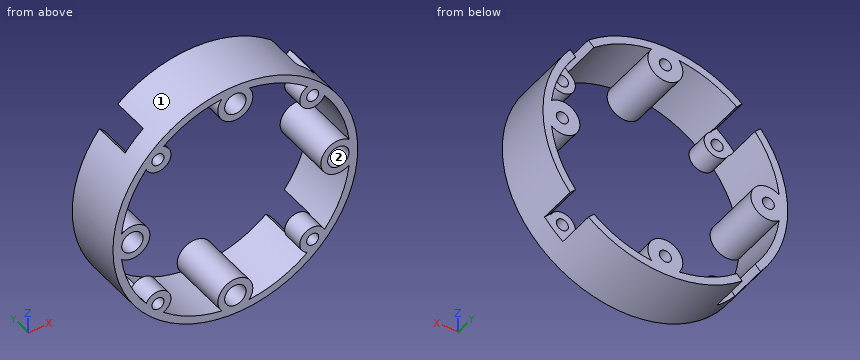
Autodesk Inventor part; units mm, degrees
ref_plane "YZ Plane" through (0, 0, 0) normal (1, 0, 0) x (0, 1, 0)
ref_plane "XZ Plane" through (0, 0, 0) normal (0, 1, 0) x (-1, 0, 0)
ref_plane "XY Plane" through (0, 0, 0) normal (0, 0, 1) x (1, 0, 0)
sketch "Sketch1" plane through (0, 0, 0) normal (0, 1, 0) x (-1, 0, 0)
  circle A0 centre (0, 0) radius 31.5
  circle A1 centre (0, 0) radius 29.5
  dimension "d0" = 63
  dimension "d1" = 59
extrude "Walls" add sketch "Sketch1" along normal blind 15.9
sketch "Sketch2" plane through (0, 0, 0) normal (0, -1, 0) x (1, 0, 0)
  circle A0 centre (0, 0) radius 31.5
  line L0 (0, -31.5) -> (0, -26.5)
  circle A1 centre (0, -26.5) radius 2.75
  circle A2 centre (0, -26.5) radius 4.5
  circle A3 centre (26.5, 0) radius 4.5
  circle A4 centre (26.5, 0) radius 2.75
  circle A5 centre (0, 26.5) radius 4.5
  circle A6 centre (0, 26.5) radius 2.75
  circle A7 centre (-26.5, 0) radius 4.5
  circle A8 centre (-26.5, 0) radius 2.75
  dimension "d4" = 5
  dimension "d5" = 5.5
  dimension "d6" = 9
  dimension "d9" = 360
extrude "Pillar holes" add sketch "Sketch2" against normal blind 15.9 contours A2 | A3 | A5 | A7
sketch "Sketch4" plane through (0, 15.9, 0) normal (0, 1, 0) x (1, 0, 0)
  point P0 (0, 0)
sketch "Sketch5" plane through (0, 0, 0) normal (0, -1, 0) x (1, 0, 0)
  point P0 (0, 0)
sketch "Sketch6" plane through (0, 15.9, 0) normal (0, 1, 0) x (1, 0, 0)
  circle A0 centre (0, 26.5) radius 2.75
  circle A1 centre (0, 26.5) radius 2.75
  circle A2 centre (0, 26.5) radius 1.55
  circle A3 centre (-26.5, 0) radius 1.55
  circle A4 centre (-26.5, 0) radius 2.75
  circle A5 centre (0, -26.5) radius 1.55
  circle A6 centre (0, -26.5) radius 2.75
  circle A7 centre (26.5, 0) radius 1.55
  circle A8 centre (26.5, 0) radius 2.75
  point P0 (0, 0)
  dimension "d20" = 3.1
  dimension "d23" = 360
extrude "Extrusion4" add sketch "Sketch6" against normal blind 8
sketch "Sketch7" plane through (0, 15.9, 0) normal (0, 1, 0) x (1, 0, 0)
  line L0 (0, 0) -> (22.2739, -22.2739)
  circle A0 centre (0, 0) radius 31.5
  line L1 (0, 0) -> (0, -31.5)
  line L2 (0, 0) -> (-22.2739, -22.2739)
  dimension "d27" = 45
ref_plane "Work Plane1" through (22.2739, 15.9, 22.2739) normal (0.7071, 0, 0.7071) x (0, 1, 0)
ref_plane "Work Plane2" through (-22.2739, 15.9, 22.2739) normal (-0.7071, 0, 0.7071) x (0, -1, 0)
sketch "Sketch17" plane through (0, 15.9, 0) normal (0, 1, 0) x (1, 0, 0)
  line L0 (0, 0) -> (-22.2739, -22.2739)
  line L1 (0, 0) -> (0, -14.1086)
  line L2 (-22.2739, -22.2739) -> (-19.9135, -19.9135)
  circle A0 centre (-19.9135, -19.9135) radius 1.55
  circle A1 centre (-19.9135, -19.9135) radius 3.338
  circle A2 centre (19.9135, -19.9135) radius 1.55
  circle A3 centre (19.9135, -19.9135) radius 3.338
  circle A4 centre (19.9135, 19.9135) radius 1.55
  circle A5 centre (19.9135, 19.9135) radius 3.338
  circle A6 centre (-19.9135, 19.9135) radius 1.55
  circle A7 centre (-19.9135, 19.9135) radius 3.338
  point P0 (22.2739, -22.2739)
  point P1 (22.2739, 22.2739)
  point P2 (-22.2739, 22.2739)
  dimension "d86" = 31.5
  dimension "d87" = 45
  dimension "d88" = 3.338
  dimension "d89" = 3.1
  dimension "d92" = 360
extrude "Extrusion13" add sketch "Sketch17" against normal blind 15.9 contours A1 L0 A0 | L0 A0 A1 | A0 L0 | L0 A0 | A2 | A3 | A4 | A5 | A6 | A7
sketch "Sketch18" plane through (0, 15.9, 0) normal (0, 1, 0) x (1, 0, 0)
  circle A0 centre (0, 0) radius 31.5
  line L0 (0, 0) -> (-22.2739, -22.2739)
  line L1 (0, 0) -> (0, -10.409)
  line L2 (-22.2739, -22.2739) -> (-19.9135, -19.9135)
  circle A1 centre (-19.9135, -19.9135) radius 1.55
  circle A2 centre (19.9135, -19.9135) radius 1.55
  circle A3 centre (19.9135, 19.9135) radius 1.55
  circle A4 centre (-19.9135, 19.9135) radius 1.55
  dimension "d96" = 45
  dimension "d97" = 3.338
  dimension "d98" = 3.1
  dimension "d101" = 360
extrude "Extrusion14" cut sketch "Sketch18" against normal blind 15.9 contours A1 L0 | L0 A1 | A2 | A3 | A4
sketch "Sketch19" plane through (0, 15.9, 0) normal (0, 1, 0) x (1, 0, 0)
  arc A0 (22.9523, -18.5322) -> (18.5322, -22.9523) centre (19.9135, -19.9135) ccw
  circle A1 centre (19.9135, -19.9135) radius 3.338
  circle A2 centre (19.9135, -19.9135) radius 1.55
  line L0 (19.9135, -19.9135) -> (17.5532, -22.2739)
  line L1 (19.9135, -19.9135) -> (22.2739, -17.5532)
  line L2 (17.5532, -22.2739) -> (19.7881, -24.5088)
  circle A3 centre (0, 0) radius 31.5
  line L3 (22.2739, -17.5532) -> (24.5088, -19.7881)
  line L4 (17.5532, -17.5532) -> (19.9135, -15.1929)
  line L5 (19.9135, -15.1929) -> (22.2739, -17.5532)
  line L6 (17.5532, -17.5532) -> (15.1929, -19.9135)
  line L7 (15.1929, -19.9135) -> (17.5532, -22.2739)
  arc A4 (19.7881, -24.5088) -> (24.5088, -19.7881) centre (0, 0) ccw
  line L8 (19.9135, 15.1929) -> (22.2739, 17.5532)
  line L9 (22.2739, 17.5532) -> (24.5088, 19.7881)
  arc A5 (24.5088, 19.7881) -> (19.7881, 24.5088) centre (0, 0) ccw
  circle A6 centre (19.9135, 19.9135) radius 3.338
  line L10 (17.5532, 17.5532) -> (15.1929, 19.9135)
  line L11 (17.5532, 17.5532) -> (19.9135, 15.1929)
  line L12 (15.1929, 19.9135) -> (17.5532, 22.2739)
  line L13 (17.5532, 22.2739) -> (19.7881, 24.5088)
  line L14 (-15.1929, 19.9135) -> (-17.5532, 22.2739)
  line L15 (-17.5532, 22.2739) -> (-19.7881, 24.5088)
  arc A7 (-19.7881, 24.5088) -> (-24.5088, 19.7881) centre (0, 0) ccw
  circle A8 centre (-19.9135, 19.9135) radius 3.338
  line L16 (-17.5532, 17.5532) -> (-19.9135, 15.1929)
  line L17 (-17.5532, 17.5532) -> (-15.1929, 19.9135)
  line L18 (-19.9135, 15.1929) -> (-22.2739, 17.5532)
  line L19 (-22.2739, 17.5532) -> (-24.5088, 19.7881)
  line L20 (-19.9135, -15.1929) -> (-22.2739, -17.5532)
  line L21 (-22.2739, -17.5532) -> (-24.5088, -19.7881)
  arc A9 (-24.5088, -19.7881) -> (-19.7881, -24.5088) centre (0, 0) ccw
  circle A10 centre (-19.9135, -19.9135) radius 3.338
  line L22 (-17.5532, -17.5532) -> (-15.1929, -19.9135)
  line L23 (-17.5532, -17.5532) -> (-19.9135, -15.1929)
  line L24 (-15.1929, -19.9135) -> (-17.5532, -22.2739)
  line L25 (-17.5532, -22.2739) -> (-19.7881, -24.5088)
  line L26 (19.9135, -15.1929) -> (24.5088, -19.7881)
  line L27 (15.1929, -19.9135) -> (19.7881, -24.5088)
  line L28 (19.9135, -15.1929) -> (15.1929, -19.9135)
  arc A11 (19.7881, -24.5088) -> (24.5088, -19.7881) centre (0, 0) ccw
  point P0 (19.7881, 24.5088)
  point P1 (-24.5088, 19.7881)
  point P2 (-19.7881, -24.5088)
  dimension "d107" = 360
extrude "Extrusion15" cut sketch "Sketch19" against normal blind 10 contours A1 A0 L0 A2 L1 | A0 L3 A3 A1 | L1 A2 L0 A0 | A3 L2 A0 A1 | L9 A6 A3 | A3 A10 L25 | A6 L13 A3 | A6 | A3 L21 A10 | A10 | L15 A8 A3 | A3 A8 L19 | A8
properties part number "cylinder"
Model file for the job. Use its own axes, mm. Face numbers are marked on the shaded views. Coordinates: 2 decimals unless noted, no trailing zeros. Order: outer loops, then holes, each group sorted by start corner. A loop starts at its lowest first (then second) coordinate and runs counter-clockwise, first axis right, second up. Notation, with made-up numbers: (-30.75, 2) -> (27.25, 2) arc R14 ccw to (27.25, 16) -> close; hole circle Ø3 at (34.5, -39.75). An arc over 180 degrees is marked (long way). Return JSON: item names as keys, results as strings. Group by question number.
Item 1: Saw through at B-B on x = 0. Write the cut outline in (y, z), then the cut area to 3 significant figures.
Item 2: Pull direction Z, two halves, no side cores. Call the marked faces 1 and 2: pulls with the +Z half, pulls with the -Z half, needs draft (parallel to the pull), parting line crosses it, or undercut.
Item 3: Wall check: line 1 along Z through (x, y) = (0, 5.5); line 2 along Z through (x, y) = (0, 10.25); line 3 along X through (y, z) = (4.5, -26.5). Give the ranges that are in metal, low to high. Write a range as [from, to].
Item 4: Saw through at D-D on x = -12. Write the cut outline in (y, z).
Item 5: Saw through at A-A on z = 0. Write the cut outline in (x, y), then the cut area to 3 significant figures.
Item 6: Saw through at C-C on y = 1.5. State how many separate pieces and enclosed holes the cut face has, then the cut area to 3 significant figures.
Item 7: Flat gauge pins, fed straight in: P1, Ø8, axis at x = 2.5, y = 5, coming from the +Z side; P2, Ø4, axis at x = -19.5, z = -19, coming from the +Y side; P3, Ø4.5, axis at x = -26.5, z = 0, coming from the -Y side; P4, Ø1, axis at x = 10, y = 6, coming from the -Z side. Where does each tip first touch, or does it go through?
Values found:
{
 "1": {"outline": "(0, -31.5) -> (15.9, -31.5) -> (15.9, -28.05) -> (7.9, -28.05) -> (7.9, -29.25) -> (0, -29.25) -> close; (0, -23.75) -> (7.9, -23.75) -> (7.9, -24.95) -> (15.9, -24.95) -> (15.9, -22) -> (0, -22) -> close; (0, 22) -> (15.9, 22) -> (15.9, 24.95) -> (7.9, 24.95) -> (7.9, 23.75) -> (0, 23.75) -> close; (0, 29.25) -> (7.9, 29.25) -> (7.9, 28.05) -> (15.9, 28.05) -> (15.9, 31.5) -> (0, 31.5) -> close", "area": "166 mm2"},
 "2": {"face 1": "parting line crosses it", "face 2": "undercut"},
 "3": {"line 1": "z = [-31.5, -29.25], [-23.75, -22], [22, 23.75], [29.25, 31.5]", "line 2": "z = [-31.5, -28.05], [-24.95, -22], [22, 24.95], [28.05, 31.5]", "line 3": "x = [-17.03, -12.96], [-4.5, -2.75], [2.75, 4.5], [12.96, 17.03]"},
 "4": {"outline": "(0, -29.12) -> (15.9, -29.12) -> (15.9, -26.95) -> (0, -26.95) -> close; (0, 26.95) -> (15.9, 26.95) -> (15.9, 29.12) -> (0, 29.12) -> close"},
 "5": {"outline": "(-31.5, 0) -> (-29.25, 0) -> (-29.25, 7.9) -> (-28.05, 7.9) -> (-28.05, 15.9) -> (-31.5, 15.9) -> close; (-24.95, 7.9) -> (-23.75, 7.9) -> (-23.75, 0) -> (-22, 0) -> (-22, 15.9) -> (-24.95, 15.9) -> close; (22, 0) -> (23.75, 0) -> (23.75, 7.9) -> (24.95, 7.9) -> (24.95, 15.9) -> (22, 15.9) -> close; (28.05, 7.9) -> (29.25, 7.9) -> (29.25, 0) -> (31.5, 0) -> (31.5, 15.9) -> (28.05, 15.9) -> close", "area": "166 mm2"},
 "6": {"separate pieces": "1", "enclosed holes": "9", "area": "586 mm2"},
 "7": {"P1": "stops at z = 31.5", "P2": "stops at y = 5.9", "P3": "stops at y = 7.9", "P4": "stops at z = -30.03"}
}
